Could you check a few things on this drawing? It's one solid part, dimensions in mm from its lowest x, y, z. A direction names the side the tool comes from. Coordinates: 2 decimals unless noted, no trailing zeros. Order: outer loops, then holes, each group sorted by start corner. A loop starts at its lowest first (then second) coordinate and runs counter-clockwise, first axis right, second up.
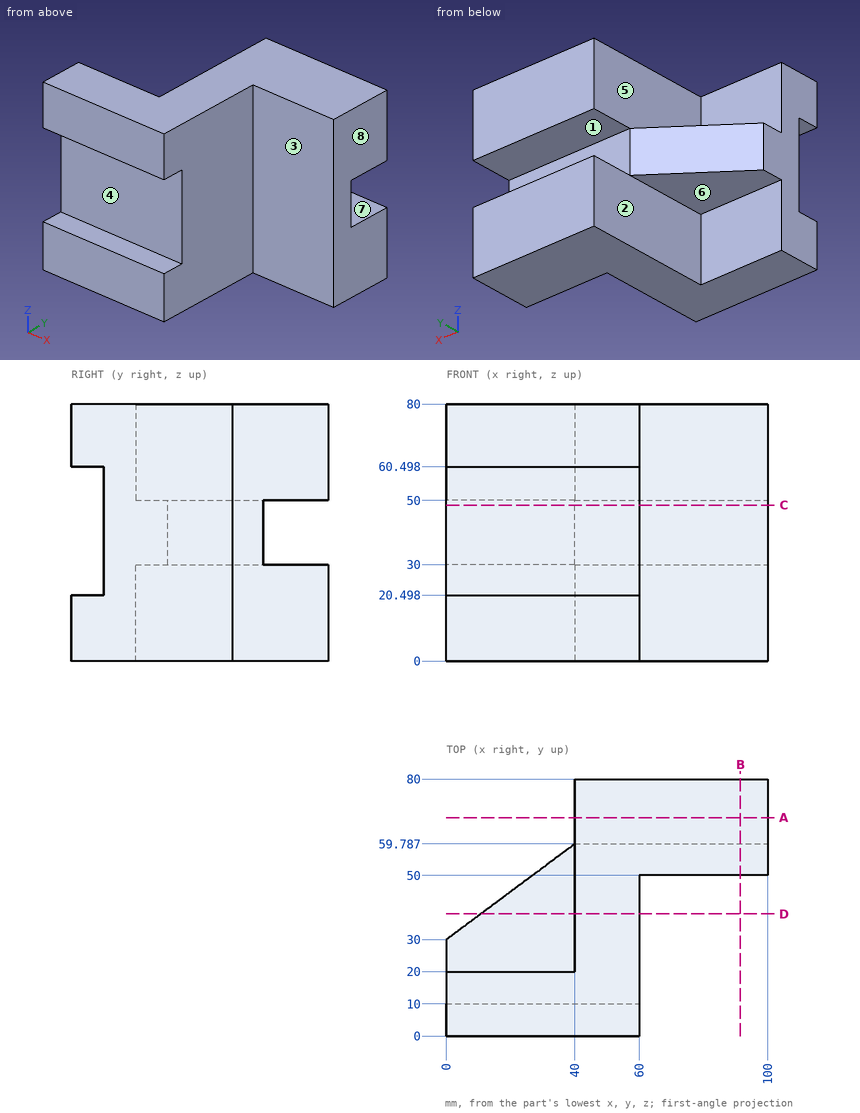
1. Please list where these lines run through material, in increasing order: probe 1 along Z at (x, y) = (83.5, 72.5); probe 2 along Y at (x, z) = (31.5, 27.5); probe 3 along Y at (x, z) = (85, 64.5).
Completed:
probe 1: z = 0 to 30, 50 to 80
probe 2: y = 10 to 20
probe 3: y = 50 to 80
2. Imagine slicing it at A-A on y = 68. Please give me the cut outline in (x, z), then the cut area to 3 significant figures.
Completed:
outline: (40, 0) - (100, 0) - (100, 30) - (40, 30) - close; (40, 50) - (100, 50) - (100, 80) - (40, 80) - close
area: 3,600 mm2
3. Imagine slicing it at C-C on z = 48.5. Please give me the cut outline in (x, y).
Completed:
outline: (0, 10) - (60, 10) - (60, 50) - (100, 50) - (100, 59.79) - (40, 59.79) - (0, 30) - close
4. On a 3-axis mill with a long thin cutter (end or side, diameter ignored), from which of +Z, -Z, +X, -X, +Y, -Y can I reach the whole of each face in a straight line? I mean the marked faces 1, 2, 3, 4 and 5. Say none if no direction works.
Completed:
face 1: +X, -X, +Y
face 2: -Z, -X, +Y
face 3: +Z, -Z, +X, -Y
face 4: +X, -X, -Y
face 5: +Z, -X, +Y
5. I'm going to push flat-ended pins straight in: pin 1 (22 mm diameter, centred on x = 61.5, y = 65.5, fed in from -Z); pin 2 (5 mm diameter, centred on y = 44, z = 45.5, fed in from +X); pin 3 (12 mm diameter, centred on x = 20.5, z = 39, fed in from -Y); pin 4 (12 mm diameter, centred on x = 13.5, y = 34.5, fed in from -Z). Where does each tip first touch, or does it pass through?
Completed:
pin 1: stops at z = 0
pin 2: stops at x = 60
pin 3: stops at y = 10
pin 4: stops at z = 30
6. Thinking about a two-plate mould opening in Z: for the marked faces 6, 7 and 8, which applies, pulls with the +Z half, pulls with the -Z half, needs draft (parallel to the pull), parting line crosses it, or undercut?
Completed:
face 6: pulls with the -Z half
face 7: undercut
face 8: needs draft
7. Imagine slicing it at D-D on y = 38. Please give me the cut outline in (x, z), then the cut area to 4 significant figures.
Completed:
outline: (10.74, 30) - (40, 30) - (40, 0) - (60, 0) - (60, 80) - (40, 80) - (40, 50) - (10.74, 50) - close
area: 2,185 mm2
8. Imagine slicing it at B-B on x = 91.5. Please give me the cut outline in (y, z), then the cut area to 3 significant figures.
Completed:
outline: (50, 0) - (80, 0) - (80, 30) - (59.79, 30) - (59.79, 50) - (80, 50) - (80, 80) - (50, 80) - close
area: 2,000 mm2
